from build123d import *

# Parameters (mm, degrees)
F0_R     = 22.5
F1_DEPTH = 3
F2_R     = 1.5
F3_DEPTH = 25


with BuildPart() as f1:
    # F0 (on Top) → F1 (new body)
    with BuildSketch(Plane.XY):
        with BuildLine():
            Line((77.5, 5), (102.377976, 5))
            ThreePointArc((102.377976, 5), (-102.5, 0), (102.377976, -5))
            Line((102.377976, -5), (77.5, -5))
            Line((77.5, -5), (77.5, 5))
        make_face()
        Circle(F0_R, mode=Mode.SUBTRACT)
    extrude(amount=F1_DEPTH)

    # F2 (on face) → F3 (cut)
    with BuildSketch(Plane.XY.offset(3)):
        with Locations((-68.34396, 37.5)):
            Circle(F2_R)
        with Locations((-39.34396, 37.5)):
            Circle(F2_R)
        with Locations((-39.34396, -37.5)):
            Circle(F2_R)
        with Locations((-68.34396, -37.5)):
            Circle(F2_R)
        with BuildLine():
            Line((-73.44097, 51.497755), (-73.247881, 51.497815))
            ThreePointArc((-73.247881, 51.497815), (-73.344427, 51.500895), (-73.44097, 51.497755))
        make_face()
        with BuildLine():
            Line((-63.344427, 51.500895), (-73.247881, 51.497815))
            Line((-73.247881, 51.497815), (-73.44097, 51.497755))
            ThreePointArc((-73.44097, 51.497755), (-74.843772, 49.977117), (-73.393472, 48.501712))
            Line((-73.393472, 48.501712), (-73.294692, 48.501704))
            Line((-73.294692, 48.501704), (-63.344082, 48.500895))
            ThreePointArc((-63.344082, 48.500895), (-61.84396, 50.001067), (-63.344427, 51.500895))
        make_face()
        with BuildLine():
            Line((-73.294692, 48.501704), (-73.393472, 48.501712))
            ThreePointArc((-73.393472, 48.501712), (-73.344082, 48.500895), (-73.294692, 48.501704))
        make_face()
        with BuildLine():
            ThreePointArc((-34.294448, 48.501712), (-32.844149, 49.977117), (-34.24695, 51.497755))
            Line((-34.24695, 51.497755), (-34.440039, 51.497815))
            Line((-34.440039, 51.497815), (-44.343494, 51.500895))
            ThreePointArc((-44.343494, 51.500895), (-45.84396, 50.001067), (-44.343838, 48.500895))
            Line((-44.343838, 48.500895), (-34.393228, 48.501704))
            Line((-34.393228, 48.501704), (-34.294448, 48.501712))
        make_face()
        with BuildLine():
            Line((-34.440039, 51.497815), (-34.24695, 51.497755))
            ThreePointArc((-34.24695, 51.497755), (-34.343494, 51.500895), (-34.440039, 51.497815))
        make_face()
        with BuildLine():
            ThreePointArc((-34.393228, 48.501704), (-34.343838, 48.500895), (-34.294448, 48.501712))
            Line((-34.294448, 48.501712), (-34.393228, 48.501704))
        make_face()
        with BuildLine():
            ThreePointArc((-34.440039, -51.497815), (-34.343494, -51.500895), (-34.24695, -51.497755))
            Line((-34.24695, -51.497755), (-34.440039, -51.497815))
        make_face()
        with BuildLine():
            Line((-34.440039, -51.497815), (-34.24695, -51.497755))
            ThreePointArc((-34.24695, -51.497755), (-32.844149, -49.977117), (-34.294448, -48.501712))
            Line((-34.294448, -48.501712), (-34.393228, -48.501704))
            Line((-34.393228, -48.501704), (-44.343838, -48.500895))
            ThreePointArc((-44.343838, -48.500895), (-45.84396, -50.001067), (-44.343494, -51.500895))
            Line((-44.343494, -51.500895), (-34.440039, -51.497815))
        make_face()
        with BuildLine():
            Line((-34.393228, -48.501704), (-34.294448, -48.501712))
            ThreePointArc((-34.294448, -48.501712), (-34.343838, -48.500895), (-34.393228, -48.501704))
        make_face()
        with BuildLine():
            ThreePointArc((-73.44097, -51.497755), (-73.344427, -51.500895), (-73.247881, -51.497815))
            Line((-73.247881, -51.497815), (-73.44097, -51.497755))
        make_face()
        with BuildLine():
            Line((-73.44097, -51.497755), (-73.247881, -51.497815))
            Line((-73.247881, -51.497815), (-63.344427, -51.500895))
            ThreePointArc((-63.344427, -51.500895), (-61.84396, -50.001067), (-63.344082, -48.500895))
            Line((-63.344082, -48.500895), (-73.294692, -48.501704))
            Line((-73.294692, -48.501704), (-73.393472, -48.501712))
            ThreePointArc((-73.393472, -48.501712), (-74.843772, -49.977117), (-73.44097, -51.497755))
        make_face()
        with BuildLine():
            ThreePointArc((-73.294692, -48.501704), (-73.344082, -48.500895), (-73.393472, -48.501712))
            Line((-73.393472, -48.501712), (-73.294692, -48.501704))
        make_face()
    extrude(amount=-F3_DEPTH, mode=Mode.SUBTRACT)


solid = f1.part
Here's how the part is built. I have some questions about the finished solid (model axes, mm). Round coordinates to 2 decimals unless told otherwise and drop trailing zeros. Write each loop counter-clockwise with the first axis right and the second up, starting at its lowest first coordinate (ties: lowest second). Pieces come first, ordered by that corner, then holes.
1. Suppose I cut it at B-B (x = 0). List the corners of the cut face in (y, z) for me.
2. Suppose I cut it at D-D (x = 68). List the corners of the cut face in (y, z) for me, and give its area (3 significant figures).
3. Suppose I cut it at C-C (y = 0). List the corners of the cut face in (x, z) for me, and give its area (3 significant figures).
4. I need wall thicknesses on L1, parallel to Y at x = -35, z = 0.35; L2, parallel to Y at x = -74.5, z = 0.25; L3, parallel to Y at x = 0, z = 0.7. Which ranges of each line are inside material? Lowest first, please.
5. Suppose I cut it at A-A (z = 1.6). State how many separate pieces and enclosed holes the cut face has, and give its area (3 significant figures).
6. If we mould it in two halves opening along X, with no side actions, what happens to faces 1 (the cylindrical face through (10.382, -19.961, 1.479)), 2 (the flat face through (-1, 24, 3)), 3 (the cylindrical face through (-102.404, 4.437, 1.479))? For each: released by +X, released by -X, zero draft, split by the parting line, or undercut.
7. Will these pins go through, and if not, where does the flat tip stop? pin 1 Ø0.9 at (y, z) = (2, 1) entering from +X; pin 2 Ø1.5 at (x, z) = (-41, 1.5) entering from +Y; pin 3 Ø1.5 at (x, z) = (-69.5, 1) entering from +Y.
Answer sheet:
1. outline: (-102.5, 0) - (-22.5, 0) - (-22.5, 3) - (-102.5, 3) - close; (22.5, 0) - (102.5, 0) - (102.5, 3) - (22.5, 3) - close
2. outline: (-76.7, 0) - (76.7, 0) - (76.7, 3) - (-76.7, 3) - close
2. area: 460 mm2
3. outline: (-102.5, 0) - (-22.5, 0) - (-22.5, 3) - (-102.5, 3) - close; (22.5, 0) - (77.5, 0) - (77.5, 3) - (22.5, 3) - close
3. area: 405 mm2
4. L1: y = -96.34 to -51.5, -48.5 to 48.5, 51.5 to 96.34
4. L2: y = -70.4 to -50.96, -49.05 to 49.05, 50.96 to 70.4
4. L3: y = -102.5 to -22.5, 22.5 to 102.5
5. separate pieces: 1
5. enclosed holes: 9
5. area: 31,000 mm2
6. face 1: undercut
6. face 2: zero draft
6. face 3: split by the parting line
7. pin 1: stops at x = 77.5
7. pin 2: stops at y = 94.27
7. pin 3: stops at y = 76.02
